```python
from build123d import *

# Parameters (mm, degrees)
F0_R     = 39.141402
F1_DEPTH = 3
F2_R     = 15.05
F3_DEPTH = 3
F5_R     = 2.3
F6_DEPTH = 3


with BuildPart() as f1:
    # F0 (on Top) → F1 (new body)
    with BuildSketch(Plane.XY):
        Circle(F0_R)
    extrude(amount=F1_DEPTH)

    # F2 (on face) → F3 (cut)
    with BuildSketch(Plane.XY.offset(3)):
        Circle(F2_R)
    extrude(amount=-F3_DEPTH, mode=Mode.SUBTRACT)

    # F5 (on face) → F6 (cut)
    with BuildSketch(Plane.XY.offset(3)):
        with Locations((15.584218, -2.272043)):
            Circle(F5_R)
        with Locations((2.653755, -15.524809)):
            Circle(F5_R)
        with Locations((-13.944715, -7.321658)):
            Circle(F5_R)
        with Locations((-11.273245, 11.001117)):
            Circle(F5_R)
        with Locations((6.977401, 14.120086)):
            Circle(F5_R)
    extrude(amount=-F6_DEPTH, mode=Mode.SUBTRACT)


solid = f1.part
```
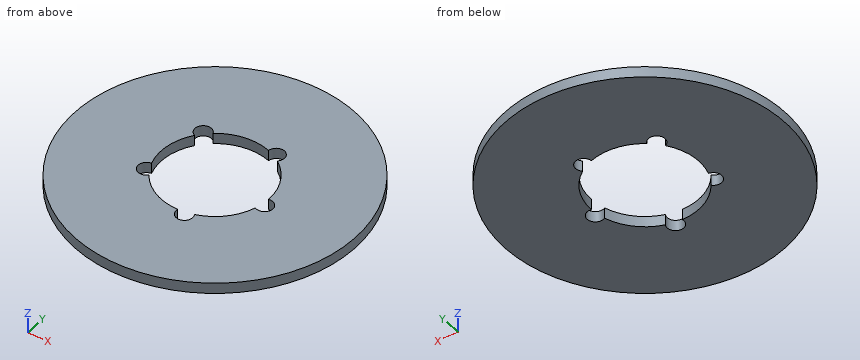
The listing builds one solid part. Answer for the finished solid, in the listing's coordinates (mm). Coordinates: 2 decimals unless noted, no trailing zeros. Write each loop counter-clockwise with the first axis right and the second up, starting at its lowest first coordinate (ties: lowest second). Pieces come first, ordered by that corner, then holes. Notation, with made-up numbers: M -33,3 L -25,3 A20 cw -25,10 Z; hole C -24,-27 d6. An arc over 180 degrees is marked long. Use a Markdown table: item, result. Add a question column.
1. Given P1, Ø7.5, axis at x = -13.94, y = -7.32, coming from the +Z side; P2, Ø1.5, axis at x = -12.5, z = 2.5, coming from the +Y side, each flat-ended and moving along its own axis, determine where each tip first touches the part or whether it passes through.
2. Section D-D (y = -25) is taken. Give the vertices of the cut face in (x, z).
3. Section C-C (z = 2.2) is taken. Give the vertices of the cut face in (x, y).
4. Section B-B (y = -16) is taken. Give the vertices of the cut face in (x, z).
5. Section A-A (x = 13.5) is taken. Give the vertices of the cut face in (y, z), plus the area to 3 significant figures.
6. Straight lines are drawn through the part: line 1 along Y through (x, z) = (9, 2.05); line 2 along Y through (x, z) = (17.5, 1.45); line 3 along X through (y, z) = (10, 2.15). For each, find the intervals that lie inside material, in ascending order. Write a range as [from, to].
Data:
| question | item | result |
|---|---|---|
| 1 | P1 | stops at z = 3 |
| 1 | P2 | stops at y = 37.34 |
| 2 | outline | M -30.12,0 L 30.12,0 L 30.12,3 L -30.12,3 Z |
| 3 | outline | C 0,0 d78.28; hole M -14.18,-5.03 A2.3 ccw long -12.2,-8.82 A15.05 ccw 0.4,-15.04 A2.3 ccw long 4.62,-14.32 A15.05 ccw 14.43,-4.26 A2.3 ccw long 15.05,-0.03 A15.05 ccw 8.51,12.41 A2.3 ccw long 4.68,14.3 A15.05 ccw -9.17,11.93 A2.3 ccw long -12.15,8.88 A15.05 ccw Z |
| 4 | outline | M -35.72,0 L 0.4,0 L 0.4,3 L -35.72,3 Z; M 4.9,0 L 35.72,0 L 35.72,3 L 4.9,3 Z |
| 5 | outline | M -36.74,0 L -6.65,0 L -6.65,3 L -36.74,3 Z; M 6.65,0 L 36.74,0 L 36.74,3 L 6.65,3 Z |
| 5 | area | 181 mm2 |
| 6 | line 1 | y = [-38.09, -12.06], [12.06, 13.03], [15.22, 38.09] |
| 6 | line 2 | y = [-35.01, -3.54], [-1, 35.01] |
| 6 | line 3 | x = [-37.84, -13.34], [11.25, 37.84] |
